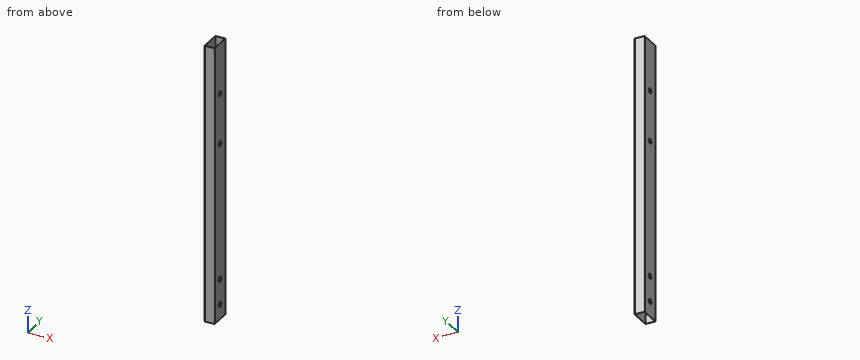
from build123d import *

# Parameters (mm, degrees)
F0_W     = 19
F0_H     = 39
F1_DEPTH = 550
F3_D     = 10
F3_DEPTH = 30
F3_TIP   = 3.0043030951


# Not quite as in the source:
# - a feature names something its author has since deleted; it is built from what else it names


with BuildPart() as f1:
    # F0 (on Top) → F1 (new body)
    with BuildSketch(Plane.XY):
        with BuildLine():
            Line((9, 20), (-9, 20))
            ThreePointArc((-9, 20), (-9.7071067812, 19.7071067812), (-10, 19))
            Line((-10, 19), (-10, -19))
            ThreePointArc((-10, -19), (-9.7071067812, -19.7071067812), (-9, -20))
            Line((-9, -20), (9, -20))
            ThreePointArc((9, -20), (9.7071067812, -19.7071067812), (10, -19))
            Line((10, -19), (10, 19))
            ThreePointArc((10, 19), (9.7071067812, 19.7071067812), (9, 20))
        make_face()
        Rectangle(F0_W, F0_H, mode=Mode.SUBTRACT)
    extrude(amount=F1_DEPTH)

    # F3
    with Locations(Plane.YZ.offset(10)):
        with Locations((0, 80), (0, 30), (0, 450), (0, 350)):
            Hole(F3_D / 2, depth=F3_DEPTH)
            with Locations((0, 0, -(F3_DEPTH + F3_TIP / 2))):  # 118° drill point
                Cone(0, F3_D / 2, F3_TIP, mode=Mode.SUBTRACT)


solid = f1.part
Source: CAD feature listing. Evaluate the final solid. Frame: model axes, mm. Round coordinates to 2 decimals unless told otherwise and drop trailing zeros. Loops run counter-clockwise (first coordinate to the right, second up) from the corner with the lowest first, then second, coordinate; pieces in that order, holes last. Notation, with made-up numbers: M 80.25,67.5 L 93.25,67.5 A23 ccw 93.25,106.5 Z; hole C 6,79.5 d4. An arc over 180 degrees is marked long. Answer as CSV lines item,"result".
Q1. Cut plane D-D (z = 309.5). Return the cut outline in (x, y), plus the area to 3 significant figures.
Verdict:
outline,"M -10,-19 A1 ccw -9,-20 L 9,-20 A1 ccw 10,-19 L 10,19 A1 ccw 9,20 L -9,20 A1 ccw -10,19 Z; hole M -9.5,-19.5 L 9.5,-19.5 L 9.5,19.5 L -9.5,19.5 Z"
area,"58.1 mm^2"
Q2. Line query: line 1 along Z through (x, y) = (-9.7, 0); line 2 along Y through (x, z) = (-1.5, 432); line 3 along X through (y, z) = (-17, 420). Output: solid intervals per line, ascending.
Verdict:
line 1,"z = 0 to 25, 35 to 75, 85 to 345, 355 to 445, 455 to 550"
line 2,"y = -20 to -19.5, 19.5 to 20"
line 3,"x = -10 to -9.5, 9.5 to 10"
Q3. Cut plane C-C (x = -1.75). Return the cut outline in (y, z), plus the area to 3 significant figures.
Verdict:
outline,"M -20,0 L -19.5,0 L -19.5,550 L -20,550 Z; M 19.5,0 L 20,0 L 20,550 L 19.5,550 Z"
area,"550 mm^2"
Q4. Cut plane B-B (z = 450). Return the cut outline in (x, y), plus the area to 3 significant figures.
Verdict:
outline,"M -10,-19 A1 ccw -9,-20 L 9,-20 A1 ccw 10,-19 L 10,-5 L 9.5,-5 L 9.5,-19.5 L -9.5,-19.5 L -9.5,-5 L -10,-5 Z; M -10,5 L -9.5,5 L -9.5,19.5 L 9.5,19.5 L 9.5,5 L 10,5 L 10,19 A1 ccw 9,20 L -9,20 A1 ccw -10,19 Z"
area,"48.1 mm^2"
Q5. Cut plane A-A (y = -12). Return the cut outline in (x, z), plus the area to 3 significant figures.
Verdict:
outline,"M -10,0 L -9.5,0 L -9.5,550 L -10,550 Z; M 9.5,0 L 10,0 L 10,550 L 9.5,550 Z"
area,"550 mm^2"
